Work out the finished part from the listing and answer in its coordinate system (mm). Face numbers are marked on the shaded views. Coordinates: 2 decimals unless noted, no trailing zeros. Write each loop counter-clockwise with the first axis right and the second up, starting at its lowest first coordinate (ties: lowest second). Pieces come first, ordered by that corner, then holes. Notation, with made-up numbers: (61, 51.5) - (116, 51.5) arc R15 ccw to (116, 61.5) - close; hole circle Ø10 at (75, 82.25). An arc over 180 degrees is marked (long way). Use one line per item in the form item = value. Start each with the question number.
Item 1: Determine the mould class of the marked faces 1, 2 and 3 for opening direction X: released by +X, released by -X, zero draft, split by the parting line, or undercut.
Item 2: A cutting plane is placed at A-A (x = 8). Write down the section's boundary in (y, z).
Item 3: A cutting plane is placed at D-D (y = -42). Write down the section's boundary in (x, z).
Item 4: A cutting plane is placed at B-B (z = 6). Give the number of separate pieces and of enclosed holes in the cut face, then the cut area to 3 significant figures.
Item 5: Given pin 1 (3 mm diameter, centred on x = -26.5, y = -15.5, fed in from +Z); pin 2 (1.5 mm diameter, centred on y = -35, z = 9.5, fed in from -X); pin 3 (6 mm diameter, centred on x = 24, z = 2.5, fed in from -Y), each flat-ended and moving along its own axis, determine where each tip first touches the part or whether it passes through.
Item 6: A cutting plane is placed at C-C (x = 38). Write down the section's boundary in (y, z).
Item 7: Consider probe 1 along Y at (x, z) = (-6.5, 5.5); probe 2 along X at (y, z) = (-15, 9.5); probe 3 along Y at (x, z) = (-15, 2). Determine where each line is inside the solid, lowest interval first.
Autodesk Inventor part; units mm, degrees
ref_plane "YZ Plane" through (0, 0, 0) normal (1, 0, 0) x (0, 1, 0)
ref_plane "XZ Plane" through (0, 0, 0) normal (0, 1, 0) x (-1, 0, 0)
ref_plane "XY Plane" through (0, 0, 0) normal (0, 0, 1) x (1, 0, 0)
sketch "Sketch1" plane through (0, 0, 0) normal (0, 0, 1) x (1, 0, 0)
  circle A0 centre (0, 0) radius 35
  point P0 (0, 35)
  point P1 (0, -35)
  dimension "d0" = 70
extrude "Extrusion1" add sketch "Sketch1" along normal blind 3
sketch "Sketch3" plane through (0, 0, 3) normal (0, 0, 1) x (1, 0, 0)
  circle A0 centre (0, 0) radius 57.5
  dimension "d8" = 115
extrude "Extrusion3" add sketch "Sketch3" along normal blind 8
sketch "Sketch7" plane through (0, 0, 11) normal (0, 0, 1) x (1, 0, 0)
  line L0 (-15, 25.9808) -> (0, 0)
  line L1 (0, 80.5) -> (0, -80.5)
  dimension "d25" = 30
  dimension "d26" = 30
hole "Hole2" at (-15, 25.9808, 11) direction (0, 0, -1) diameter 3.4 end through all counterbore diameter 6.5 counterbore depth 3.4
pattern_circular "Circular Pattern1" count 8 over 360 about axis through (0, 0, -10) along (0, 0, 1) of "Hole2"
sketch "Sketch12" plane through (0, 0, 11) normal (0, 0, 1) x (1, 0, 0)
  line L0 (-12.4233, 46.3644) -> (0, 0)
  line L1 (0, 80.5) -> (0, -80.5)
  dimension "d77" = 15
  dimension "d78" = 48
hole "Hole6" at (-12.4233, 46.3644, 11) direction (0, 0, -1) diameter 3.2 end through all
pattern_circular "Circular Pattern2" count 12 over 360 about axis through (0, 0, -10) along (0, 0, 1) of "Hole6"
sketch "Sketch8" plane through (0, 0, 11) normal (0, 0, 1) x (1, 0, 0)
  circle A0 centre (0, 0) radius 20
  dimension "d89" = 40
extrude "Extrusion4" cut sketch "Sketch8" against normal through all
equation "\"d79\" = M3_adjustable"
equation "\"bearing_61807_inner\" = 35"
equation "\"bearing_61807_outer\" = 47.1"
equation "\"bearing_61814_outer\" = 90.1"
equation "\"M3_adjustable\" = 3.2"
properties part number "201-"
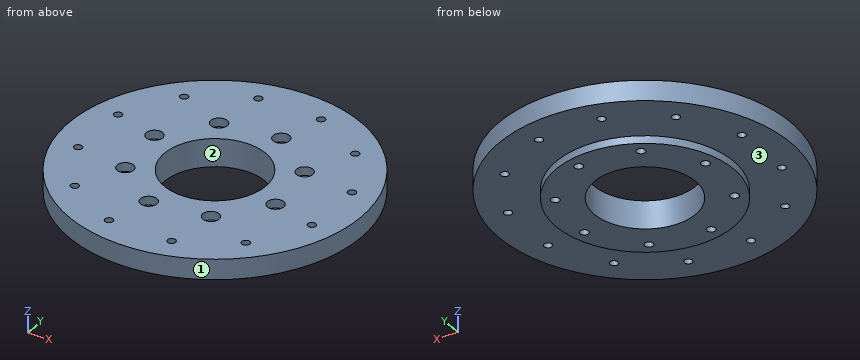
Answer:
q1.face_1 = split by the parting line
q1.face_2 = undercut
q1.face_3 = zero draft
q2.outline = (-56.94, 3) - (-34.07, 3) - (-34.07, 0) - (-18.33, 0) - (-18.33, 11) - (-56.94, 11) - close; (18.33, 0) - (27.29, 0) - (27.29, 7.6) - (25.74, 7.6) - (25.74, 11) - (18.33, 11) - close; (30.66, 0) - (34.07, 0) - (34.07, 3) - (56.94, 3) - (56.94, 11) - (32.22, 11) - (32.22, 7.6) - (30.66, 7.6) - close
q3.outline = (-39.27, 3) - (39.27, 3) - (39.27, 11) - (-39.27, 11) - close
q4.separate_pieces = 1
q4.enclosed_holes = 21
q4.area = 8,960 mm²
q5.pin_1 = 7.6
q5.pin_2 = -46.19
q5.pin_3 = -53.51
q6.outline = (-43.15, 3) - (43.15, 3) - (43.15, 11) - (-43.15, 11) - close
q7.probe_1 = -57.13 to -30.11, -27.84 to -18.91, 18.91 to 57.13
q7.probe_2 = -55.51 to -29.23, -22.73 to -13.23, 13.23 to 55.51
q7.probe_3 = -31.62 to -13.23, 13.23 to 24.28, 27.68 to 31.62
